Source: CAD feature listing. Evaluate the final solid. Frame: model axes, mm. A direction names the side the tool comes from. Coordinates: 2 decimals unless noted, no trailing zeros. Order: outer loops, then holes, each group sorted by start corner. A loop starts at its lowest first (then second) coordinate and runs counter-clockwise, first axis right, second up.
```python
from build123d import *

# Parameters (mm, degrees)
BOSS_EXTRUDE1_DEPTH = 6
BOSS_EXTRUDE2_DEPTH = 2
FILLET1_R           = 1
BOSS_EXTRUDE3_DEPTH = 6.75
FILLET2_R           = 0.5
SKETCH6_R           = 0.65
CUT_EXTRUDE1_DEPTH  = 2.5
FILLET3_R           = 0.5
SKETCH8_W           = 3.5
SKETCH8_H           = 4.75
CUT_EXTRUDE2_DEPTH  = 1
SKETCH9_W           = 8.81
SKETCH9_H           = 0.125
CUT_EXTRUDE3_DEPTH  = 15.397730865
SKETCH10_W          = 3.5
SKETCH10_H          = 2
CUT_EXTRUDE4_DEPTH  = 0.1


with BuildPart() as part:
    # Sketch2 → Boss-Extrude1 (new, symmetric)
    with BuildSketch(Plane.XY):
        with BuildLine():
            Line((4.405, 0.975), (-0.883991622, 0.975))
            ThreePointArc((-0.883991622, 0.975), (-2.787934898, 0.598310502), (-4.405, -0.475))
            Line((-4.405, -0.475), (-4.405, -0.975))
            Line((-4.405, -0.975), (4.405, -0.975))
            Line((4.405, -0.975), (4.405, 0.975))
        make_face()
    extrude(amount=BOSS_EXTRUDE1_DEPTH, both=True)

    # Sketch3 → Boss-Extrude2 (add, symmetric)
    with BuildSketch(Plane.XY):
        with BuildLine():
            ThreePointArc((-1.155, 2.375), (-2.894244197, 1.987819633), (-4.305, 0.899404694))
            Line((-4.305, 0.899404694), (-4.305, -0.37853573))
            ThreePointArc((-4.305, -0.37853573), (-2.723513115, 0.624318302), (-0.883991622, 0.975))
            Line((-0.883991622, 0.975), (0.795, 0.975))
            Line((0.795, 0.975), (0.795, 2.375))
            Line((0.795, 2.375), (-1.155, 2.375))
        make_face()
    extrude(amount=BOSS_EXTRUDE2_DEPTH, both=True)

    # Fillet1
    fillet1_edges = [part.edges().sort_by_distance(p)[0] for p in [
        (0.795, 1.675, -2),
        (-4.305, 0.260434482, -2),
        (0.795, 1.675, 2),
        (-4.305, 0.260434482, 2),
    ]]
    fillet(fillet1_edges, radius=FILLET1_R)

    # Cut-Sweep1: sweep along a path in Sketch4
    with BuildLine(Plane.XY.offset(2)) as cut_sweep1_path:
        Line((0.795, 2.375), (-0.205, 2.375))
        Line((-0.205, 2.375), (-1.155, 2.375))
        ThreePointArc((-1.155, 2.375), (-2.27228554, 2.219828643), (-3.305, 1.766060011))
        ThreePointArc((-3.305, 1.766060011), (-3.840195125, 1.373342644), (-4.305, 0.899404694))
    # Sketch5 → Cut-Sweep1 (sweep, cut)
    with BuildSketch(Plane(origin=(0.795, 0, 0), x_dir=(0, 0, -1), z_dir=(1, 0, 0))):
        Polygon((-1.815, 2.375), (-1.665, 2.225), (-1.515, 2.375), (-1.335, 2.375), (-1.185, 2.225), (-1.035, 2.375), (-0.855, 2.375), (-0.705, 2.225), (-0.555, 2.375), (-0.375, 2.375), (-0.375, 2.225), (0.375, 2.225), (0.375, 2.375), (0.555, 2.375), (0.705, 2.225), (0.855, 2.375), (1.035, 2.375), (1.185, 2.225), (1.335, 2.375), (1.515, 2.375), (1.665, 2.225), (1.815, 2.375), (1.815, 2.475), (-1.815, 2.475), align=None)
    sweep(path=cut_sweep1_path.line, mode=Mode.SUBTRACT)

    # Sketch7 → Boss-Extrude3 (add, symmetric)
    with BuildSketch(Plane.XY):
        with BuildLine():
            Line((4.405, -0.975), (4.405, 0.975))
            Line((4.405, 0.975), (-0.883991622, 0.975))
            ThreePointArc((-0.883991622, 0.975), (-2.167505893, 0.807451874), (-3.365, 0.316036446))
            Line((-3.365, 0.316036446), (-3.365, -0.975))
            Line((-3.365, -0.975), (4.405, -0.975))
        make_face()
    extrude(amount=BOSS_EXTRUDE3_DEPTH, both=True)

    # Fillet2
    fillet2_edges = [part.edges().sort_by_distance(p)[0] for p in [
        (-4.405, -0.725, 6),
        (4.405, 0, -6.75),
        (-3.365, -0.329481777, -6.75),
        (4.405, 0, 6.75),
        (-3.365, -0.329481777, 6.75),
        (-4.405, -0.725, -6),
    ]]
    fillet(fillet2_edges, radius=FILLET2_R)

    # Sketch6 → Cut-Extrude1 (cut)
    with BuildSketch(Plane(origin=(4.405, 0, 0), x_dir=(0, 0, -1), z_dir=(1, 0, 0))):
        with Locations((0, 0.125)):
            Circle(SKETCH6_R)
    extrude(amount=-CUT_EXTRUDE1_DEPTH, mode=Mode.SUBTRACT)

    # Fillet3
    fillet3_edges = [part.edges().sort_by_distance(p)[0] for p in [
        (-3.635, -0.975, 6),
        (-4.258553391, -0.975, 5.853553391),
        (-3.635, -0.975, -6),
        (-4.258553391, -0.975, -5.853553391),
        (-4.405, -0.975, 0),
    ]]
    fillet(fillet3_edges, radius=FILLET3_R - 0.0001)  # a hair under: the kernel refuses the full size

    # Sketch8 → Cut-Extrude2 (cut)
    with BuildSketch(Plane.XZ.offset(0.975)):
        with Locations((2.655, -3.375)):
            Rectangle(SKETCH8_W, SKETCH8_H)
        with Locations((2.655, 3.375)):
            Rectangle(SKETCH8_W, SKETCH8_H)
    extrude(amount=-CUT_EXTRUDE2_DEPTH, mode=Mode.SUBTRACT)

    # Sketch9 → Cut-Extrude3 (cut, through all)
    with BuildSketch(Plane.XY.offset(6.75)):
        with Locations((0, -0.9125)):
            Rectangle(SKETCH9_W, SKETCH9_H)
    extrude(amount=-CUT_EXTRUDE3_DEPTH, mode=Mode.SUBTRACT)

    # Sketch10 → Cut-Extrude4 (cut)
    with BuildSketch(Plane.XZ.offset(0.85)):
        with Locations((2.655, 0)):
            Rectangle(SKETCH10_W, SKETCH10_H)
    extrude(amount=-CUT_EXTRUDE4_DEPTH, mode=Mode.SUBTRACT)


solid = part.part
```
Q1. Set-up query: faces 4 (the cylindrical face through (-4.004, 0.679, -1.715)), 5 (the cylindrical face through (-4.004, 0.679, 1.715)), 6 (the flat face through (3, 0.025, 3)), 7 (the cylindrical face through (0.51, 1.68, -1.7)), 8 (the flat face through (-4.305, 0, 0)). Return all of +Z, -Z, +X, -X, +Y, -Y with unobstructed straight access to the full face (end or side cutting, diameter ignored); none if empty.
Solutions:
face 4: -Z, -X, +Y
face 5: +Z, -X, +Y
face 6: +X, -Y
face 7: -Z, +X, +Y
face 8: +Z, -Z, -X, +Y
Q2. Section query B-B on x = 3.25. Output: boundary loops of the cut face in (y, z) (3 decimals).
Solutions:
outline: (-0.85, -6.75) - (0.975, -6.75) - (0.975, 6.75) - (-0.85, 6.75) - (-0.85, 5.75) - (0.025, 5.75) - (0.025, 1) - (-0.75, 1) - (-0.75, -1) - (0.025, -1) - (0.025, -5.75) - (-0.85, -5.75) - close; hole circle Ø1.3 at (0.125, 0)
Q3. Material intervals for line 1 along Y through (x, z) = (3.5, 0) (3 decimals); line 2 along Z through (x, y) = (2.75, -0.7); line 3 along Z through (x, y) = (3.5, -0.15), sorted ascending.
Solutions:
line 1: y = -0.75 to -0.525, 0.775 to 0.975
line 2: z = -6.75 to -5.75, -1 to 1, 5.75 to 6.75
line 3: z = -6.75 to -5.75, -1 to -0.59, 0.59 to 1, 5.75 to 6.75
Q4. Pin query (flat end, axial travel): P1, Ø0.6, axis at y = 0, z = 0, coming from the +X side (3 decimals); P2, Ø1.6, axis at x = -1.5, y = 1, coming from the +Z side; P3, Ø1.7, axis at x = 3, z = 3.5, coming from the -Y side (3 decimals); P4, Ø3, axis at x = 2.5, z = -4, coming from the +Y side (3 decimals). Return the tip coordinate at first contact, or that it passes through.
Solutions:
P1: stops at x = 1.905
P2: stops at z = 6.75
P3: stops at y = 0.025
P4: stops at y = 0.975
Q5. Pull-direction query (Z, two-part tool) for faces 1 (the flat face through (2, 0.975, 0)), 2 (the flat face through (2.6, -0.4, 5.75)), 3 (the flat face through (0, 0, -6.75)); classes: pulls with the +Z half, pulls with the -Z half, needs draft (parallel to the pull), parting line crosses it, or undercut.
Solutions:
face 1: needs draft
face 2: undercut
face 3: pulls with the -Z half
